from build123d import *

# Parameters (mm, degrees)
SKETCH1_W               = 241.3
SKETCH1_H               = 50.8
BOSS_EXTRUDE1_DEPTH     = 12.7
F_1_4_20_TAPPED_HOLE2_D = 5.1054
F_1_2_CLEARANCE_HOLE1_D = 13.49248


with BuildPart() as part:
    # Sketch1 → Boss-Extrude1 (new body)
    with BuildSketch(Plane(origin=(0, 0, 0), x_dir=(1, 0, 0), z_dir=(0, 1, 0))):
        Rectangle(SKETCH1_W, SKETCH1_H)
    extrude(amount=BOSS_EXTRUDE1_DEPTH)

    # 1/4-20 Tapped Hole2 (through all)
    with Locations(Plane(origin=(0, 12.7, 0), x_dir=(1, 0, 0), z_dir=(0, 1, 0))):
        with Locations((60.325, -12.7), (-34.925, -12.7), (-60.325, -12.7), (-60.325, 12.7), (-34.925, 12.7), (34.925, 12.7), (60.325, 12.7), (34.925, -12.7)):
            Hole(F_1_4_20_TAPPED_HOLE2_D / 2)

    # 1/2 Clearance Hole1 (through all)
    with Locations(Plane(origin=(0, 12.7, 0), x_dir=(1, 0, 0), z_dir=(0, 1, 0))):
        with Locations((-107.95, 0), (107.95, 0)):
            Hole(F_1_2_CLEARANCE_HOLE1_D / 2)


solid = part.part
For this review, take the finished solid that the model builds, in its own axes (mm). Give positions to 0.01 mm unless a question says otherwise; leave off trailing zeros. Loops run counter-clockwise (first coordinate to the right, second up) from the corner with the lowest first, then second, coordinate; pieces in that order, holes last. Notation, with made-up numbers: M 29.5,74 L 73.5,74 A20 cw 73.5,91 Z; hole C 51.5,54 d5. An arc over 180 degrees is marked long. Answer as a JSON object with one key per item and string values. Group by question number.
Q1. Mouldability with a two-part tool opening along X and no side actions: class faces 1 (the flat face through (-2, 0, 0)), 2 (the flat face through (120.65, 6, 0)), 3 (the cylindrical face through (101.515, 6.261, -2.026)) as +X half, -X half, draft (parallel to the pull), parting line (faces both ways), or undercut.
Q2. Add section C-C on z = 12.7. Give the boundary of the cut face in (x, y), and give its area (3 significant figures).
Q3. Insertion check: P1, Ø1, axis at x = 43.5, z = -15.5, coming from the -Y side. The pin has a flat end and moves straight along its axis. Give the tip position at first contact, or say it passes through.
Q4. Add section B-B on y = 9.75. Give the number of separate pieces and of enclosed holes in the cut face, and give its area (3 significant figures).
Q5. For probe 1 along X at (y, z) = (8.75, -12.5); probe 2 along Z at (x, y) = (-35.5, 5); probe 3 along Z at (x, y) = (-107.95, 4.75), list the stretches that pass through material, from the lowest coordinate up. Write a range as [from, to].
Q6. Add section A-A on z = 0. Give the boundary of the cut face in (x, y).
Checked values:
{
 "1": {"face 1": "draft", "face 2": "+X half", "face 3": "undercut"},
 "2": {"outline": "M -120.65,0 L -62.88,0 L -62.88,12.7 L -120.65,12.7 Z; M -57.77,0 L -37.48,0 L -37.48,12.7 L -57.77,12.7 Z; M -32.37,0 L 32.37,0 L 32.37,12.7 L -32.37,12.7 Z; M 37.48,0 L 57.77,0 L 57.77,12.7 L 37.48,12.7 Z; M 62.88,0 L 120.65,0 L 120.65,12.7 L 62.88,12.7 Z", "area": "2,810 mm²"},
 "3": {"P1": "y = 0"},
 "4": {"separate pieces": "1", "enclosed holes": "10", "area": "11,800 mm²"},
 "5": {"probe 1": "[-120.65, -62.87], [-57.78, -37.47], [-32.38, 32.38], [37.47, 57.78], [62.87, 120.65]", "probe 2": "[-25.4, -15.19], [-10.21, 10.21], [15.19, 25.4]", "probe 3": "[-25.4, -6.75], [6.75, 25.4]"},
 "6": {"outline": "M -120.65,0 L -114.7,0 L -114.7,12.7 L -120.65,12.7 Z; M -101.2,0 L 101.2,0 L 101.2,12.7 L -101.2,12.7 Z; M 114.7,0 L 120.65,0 L 120.65,12.7 L 114.7,12.7 Z"}
}
